```python
from build123d import *

# Parameters (mm, degrees)
F0_W     = 63.5
F0_H     = 63.5
F1_DEPTH = 63.5
F2_R     = 31.75
F3_DEPTH = 127.001
F4_R     = 31.75
F5_DEPTH = 127.001
F6_R     = 31.75
F7_DEPTH = 127.001


with BuildPart() as f1:
    # F0 (on Top) → F1 (new body, symmetric)
    with BuildSketch(Plane.XY):
        with Locations((-31.75, 31.75)):
            Rectangle(F0_W, F0_H)
        with Locations((-31.75, -31.75)):
            Rectangle(F0_W, F0_H)
        with Locations((31.75, -31.75)):
            Rectangle(F0_W, F0_H)
        with Locations((31.75, 31.75)):
            Rectangle(F0_W, F0_H)
    extrude(amount=F1_DEPTH, both=True)

    # F2 (on face) → F3 (cut, through all)
    with BuildSketch(Plane.YZ.offset(63.5)):
        Circle(F2_R)
    extrude(amount=-F3_DEPTH, mode=Mode.SUBTRACT)

    # F4 (on face) → F5 (cut, through all)
    with BuildSketch(Plane.XZ.offset(63.5)):
        Circle(F4_R)
    extrude(amount=-F5_DEPTH, mode=Mode.SUBTRACT)

    # F6 (on face) → F7 (cut, through all)
    with BuildSketch(Plane.XY.offset(63.5)):
        Circle(F6_R)
    extrude(amount=-F7_DEPTH, mode=Mode.SUBTRACT)


solid = f1.part
```
Geometry check sheet. Reference: the model listing, model coordinates, mm. Round coordinates to 2 decimals unless told otherwise and drop trailing zeros. Loops run counter-clockwise (first coordinate to the right, second up) from the corner with the lowest first, then second, coordinate; pieces in that order, holes last. Notation, with made-up numbers: M -20.5,72 L 2.5,72 A17 ccw 2.5,89 Z; hole C -4,74.5 d7. An arc over 180 degrees is marked long. Return JSON: item names as keys, results as strings. Group by question number.
(1) Scan lines: line 1 along Z through (x, y) = (0, -41); line 2 along X through (y, z) = (19.5, 40). Record each from-to range of solid material in increasing order. Write a range as [from, to].
(2) Section check A-A, the plane z = 0. Enter the section's corners in (x, y).
(3) Mould release check, pull along Y, two halves, no side actions. Record for faces 1 (the face through (-15, 29, -63.5)), 2 (the face through (15, 63.5, 29)), 3 (the face through (-47.25, -23.4, 21.46)): pulls with the +Y half, pulls with the -Y half, needs draft (parallel to the pull), parting line crosses it, or undercut.
(4) Section check C-C, the plane z = -56. Enter the section's corners in (x, y), and give its area (3 significant figures).
Data:
{
 "1": {"line 1": "[-63.5, -31.75], [31.75, 63.5]", "line 2": "[-63.5, -25.06], [25.06, 63.5]"},
 "2": {"outline": "M -63.5,-63.5 L -31.75,-63.5 L -31.75,-31.75 L -63.5,-31.75 Z; M -63.5,31.75 L -31.75,31.75 L -31.75,63.5 L -63.5,63.5 Z; M 31.75,-63.5 L 63.5,-63.5 L 63.5,-31.75 L 31.75,-31.75 Z; M 31.75,31.75 L 63.5,31.75 L 63.5,63.5 L 31.75,63.5 Z"},
 "3": {"face 1": "needs draft", "face 2": "pulls with the +Y half", "face 3": "undercut"},
 "4": {"outline": "M -63.5,-63.5 L 63.5,-63.5 L 63.5,63.5 L -63.5,63.5 Z; hole C 0,0 d63.5", "area": "13,000 mm²"}
}
